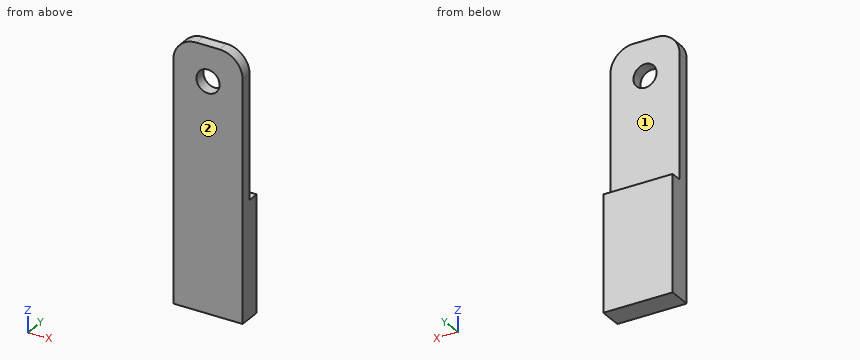
from build123d import *

# Parameters (mm, degrees)
F0_W     = 30
F0_H     = 113.08
F0_R     = 5
F1_DEPTH = 5
F2_R     = 10
F3_W     = 30
F3_H     = 50
F4_DEPTH = 5


with BuildPart() as f1:
    # F0 (on Front) → F1 (new body)
    with BuildSketch(Plane.XZ):
        Rectangle(F0_W, F0_H)
        with Locations((0, 41.54)):
            Circle(F0_R, mode=Mode.SUBTRACT)
    extrude(amount=F1_DEPTH)

    # F2
    f2_edges = [f1.edges().sort_by_distance(p)[0] for p in [
        (15, -2.5, 56.54),
        (-15, -2.5, 56.54),
    ]]
    fillet(f2_edges, radius=F2_R)

    # F3 (on face) → F4 (join)
    with BuildSketch(Plane(origin=(0, 0, 0), x_dir=(-1, 0, 0), z_dir=(0, 1, 0))):
        with Locations((0, -31.54)):
            Rectangle(F3_W, F3_H)
    extrude(amount=F4_DEPTH)


solid = f1.part
The listing builds one solid part. Answer for the finished solid, in the listing's coordinates (mm). Face numbers are marked on the shaded views. A direction names the side the tool comes from. Give positions to 0.01 mm unless a question says otherwise; leave off trailing zeros. Loops run counter-clockwise (first coordinate to the right, second up) from the corner with the lowest first, then second, coordinate; pieces in that order, holes last.
Item 1: A cutting plane is placed at B-B (y = -1.25). Give the vertices of the cut face in (x, z).
Derived:
outline: (-15, -56.54) - (15, -56.54) - (15, 46.54) arc R10 ccw to (5, 56.54) - (-5, 56.54) arc R10 ccw to (-15, 46.54) - close; hole circle Ø10 at (0, 41.54)
Item 2: Each of these flat-tipped pins is pushed along its axis until it touches: pin 1 Ø1.5 at (x, y) = (-9, -3) entering from +Z; pin 2 Ø15 at (x, z) = (2.5, 37.5) entering from +Y; pin 3 Ø6 at (x, y) = (0.5, 3.5) entering from +Z; pin 4 Ø5.5 at (x, y) = (4.5, 1.5) entering from +Z. Where does it stop, or does it pass through?
Derived:
pin 1: stops at z = 56
pin 2: stops at y = 0
pin 3: stops at z = -6.54
pin 4: stops at z = 56.54
Item 3: A cutting plane is placed at C-C (x = 0). Give the vertices of the cut face in (y, z).
Derived:
outline: (-5, -56.54) - (5, -56.54) - (5, -6.54) - (0, -6.54) - (0, 36.54) - (-5, 36.54) - close; (-5, 46.54) - (0, 46.54) - (0, 56.54) - (-5, 56.54) - close
Item 4: A cutting plane is placed at D-D (z = 9). Give the vertices of the cut face in (x, y), then the cut area to 3 significant figures.
Derived:
outline: (-15, -5) - (15, -5) - (15, 0) - (-15, 0) - close
area: 150 mm2
Item 5: A cutting plane is placed at A-A (z = 41.54). Give the vertices of the cut face in (x, y), then the cut area to 3 significant figures.
Derived:
outline: (-15, -5) - (-5, -5) - (-5, 0) - (-15, 0) - close; (5, -5) - (15, -5) - (15, 0) - (5, 0) - close
area: 100 mm2
Item 6: Find the intervals of material crossed by line 1 along Z through (x, y) = (0, -2); line 2 along Y through (x, z) = (10.5, 10); line 3 along Z through (x, y) = (9.5, 3.75), in increasing order.
Derived:
line 1: z = -56.54 to 36.54, 46.54 to 56.54
line 2: y = -5 to 0
line 3: z = -56.54 to -6.54
Item 7: A tool of negligible diameter and unlimited length cuts with its end or side. For the marked faces 1 and 2, from which of +Z, -Z, +X, -X, +Y, -Y can it reach the whole face along a straight path? Write none if from no direction.
Derived:
face 1: +Z, +X, -X, +Y
face 2: +Z, -Z, +X, -X, -Y
